from build123d import *

# Parameters (mm, degrees)
SKETCH1_R         = 76.2
ROUND_PLATE_DEPTH = 12.7
SKETCH2_R         = 12.7
CENTRE_BORE_DEPTH = 109.508847566
SKETCH3_R         = 3.81
SEED_HOLE_DEPTH   = 109.508847566


with BuildPart() as part:
    # Sketch1 → round_plate (new body)
    with BuildSketch(Plane.XY):
        Circle(SKETCH1_R)
    extrude(amount=ROUND_PLATE_DEPTH)

    # Sketch2 → centre_bore (cut, through all)
    with BuildSketch(Plane.XY):
        Circle(SKETCH2_R)
    extrude(amount=CENTRE_BORE_DEPTH, mode=Mode.SUBTRACT)

    # Sketch3 → seed_hole (cut, through all)
    with BuildSketch(Plane.XY):
        with Locations((50.8, 0)):
            Circle(SKETCH3_R)
    extrude(amount=SEED_HOLE_DEPTH, mode=Mode.SUBTRACT)


solid = part.part
Design review of the part built by this model. Coordinates are the model's own, in mm. Coordinates: 2 decimals unless noted, no trailing zeros. Loops run counter-clockwise (first coordinate to the right, second up) from the corner with the lowest first, then second, coordinate; pieces in that order, holes last. Notation, with made-up numbers: (25, -37) -> (32, -37) arc R22 cw to (32, -19) -> close; hole circle Ø1 at (7.25, 15.5). An arc over 180 degrees is marked (long way). Use a Markdown table: item, result. Add a question column.
Item 1: Clearance check with flat-ended pins moving along their axes: P1, Ø15, axis at x = 0, y = 0, coming from the +Z side; P2, Ø6, axis at x = -42.5, z = 1.5, coming from the +Y side; P3, Ø1, axis at y = 52, z = 3, coming from the -X side; P4, Ø2, axis at x = -38, z = 10, coming from the +Y side. State where each tip first meets the part, or that it passes through.
Item 2: We need section B-B, the plane y = 0. Write out the cut boundary in (x, z), and give its area (3 significant figures).
Item 3: We need section D-D, the plane x = 50.8. Write out the cut boundary in (y, z), and give its area (3 significant figures).
Item 4: The part is to be moulded in two halves that separate along X. For faces 1 (the flat face through (-1, -16, 0)), 2 (the cylindrical face through (-60.47, -46.367, 6.261)), 3 (the cylindrical face through (46.994, 0.168, 6.261)), say which applies: +X half, -X half, draft (parallel to the pull), parting line (faces both ways), or undercut.
Item 5: We need section A-A, the plane x = 0. Write out the cut boundary in (y, z).
Item 6: Wall thickness on L1, parallel to Y at x = 0, z = 9.5; L2, parallel to Y at x = -8.5, z = 8; L3, parallel to X at y = -9, z = 1.25: over which ranges is each line inside the solid? List them lowest first. Write a range as from..to.
Item 7: We need section C-C, the plane z = 2.25. Write out the cut boundary in (x, y), and give its area (3 significant figures).
Numbers:
| question | item | result |
|---|---|---|
| 1 | P1 | passes through |
| 1 | P2 | stops at y = 65.16 |
| 1 | P3 | stops at x = -56.16 |
| 1 | P4 | stops at y = 66.61 |
| 2 | outline | (-76.2, 0) -> (-12.7, 0) -> (-12.7, 12.7) -> (-76.2, 12.7) -> close; (12.7, 0) -> (46.99, 0) -> (46.99, 12.7) -> (12.7, 12.7) -> close; (54.61, 0) -> (76.2, 0) -> (76.2, 12.7) -> (54.61, 12.7) -> close |
| 2 | area | 1,520 mm^2 |
| 3 | outline | (-56.8, 0) -> (-3.81, 0) -> (-3.81, 12.7) -> (-56.8, 12.7) -> close; (3.81, 0) -> (56.8, 0) -> (56.8, 12.7) -> (3.81, 12.7) -> close |
| 3 | area | 1,350 mm^2 |
| 4 | face 1 | draft |
| 4 | face 2 | parting line |
| 4 | face 3 | undercut |
| 5 | outline | (-76.2, 0) -> (-12.7, 0) -> (-12.7, 12.7) -> (-76.2, 12.7) -> close; (12.7, 0) -> (76.2, 0) -> (76.2, 12.7) -> (12.7, 12.7) -> close |
| 6 | L1 | y = -76.2..-12.7, 12.7..76.2 |
| 6 | L2 | y = -75.72..-9.44, 9.44..75.72 |
| 6 | L3 | x = -75.67..-8.96, 8.96..75.67 |
| 7 | outline | circle Ø152.4 at (0, 0); hole circle Ø25.4 at (0, 0); hole circle Ø7.62 at (50.8, 0) |
| 7 | area | 17,700 mm^2 |
